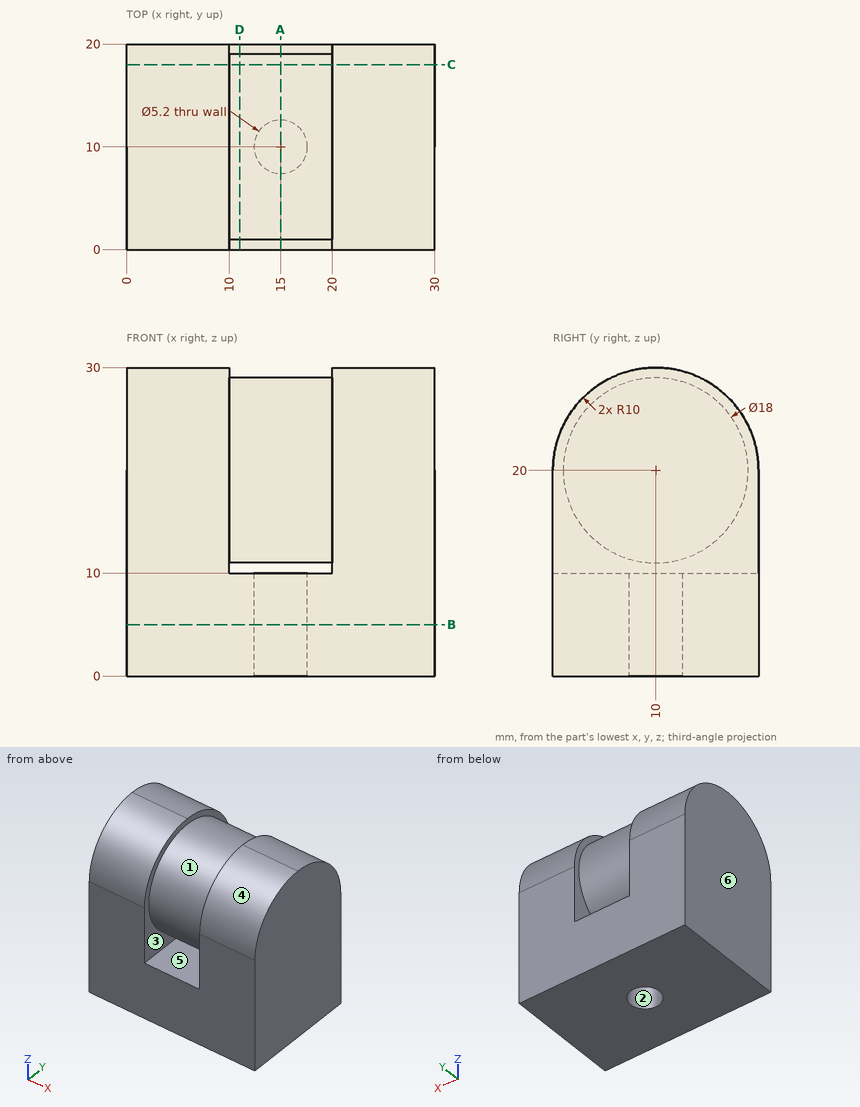
Answer from the drawing. Dimensions are ordinates in mm from the lowest x, y and z of the part. A direction names the side the tool comes from. Coordinates: 2 decimals unless noted, no trailing zeros. Order: outer loops, then holes, each group sorted by start corner. A loop starts at its lowest first (then second) coordinate and runs counter-clockwise, first axis right, second up. Notation, with made-up numbers: (46.5, 48) - (103.5, 48) arc R23 ccw to (103.5, 80) - close; hole circle Ø8 at (35.25, 6). An arc over 180 degrees is marked (long way). Use one line per item in the form item = value.
(1) Section D-D, the plane x = 11 is taken. Give the vertices of the cut face in (y, z), then the cut area to 3 significant figures.
Computed values:
outline = (0, 0) - (20, 0) - (20, 10) - (0, 10) - close; circle Ø18 at (10, 20)
area = 454 mm²
(2) Section C-C, the plane y = 18 is taken. Give the vertices of the cut face in (x, z), then the cut area to 3 significant figures.
Computed values:
outline = (0, 0) - (30, 0) - (30, 26) - (20, 26) - (20, 24.12) - (10, 24.12) - (10, 26) - (0, 26) - close; hole (10, 10) - (20, 10) - (20, 15.88) - (10, 15.88) - close
area = 702 mm²
(3) Section B-B, the plane z = 5 is taken. Give the vertices of the cut face in (x, y).
Computed values:
outline = (0, 0) - (30, 0) - (30, 20) - (0, 20) - close; hole circle Ø5.2 at (15, 10)
(4) Which of the six approach directions +Z, -Z, +X, -X, +Y, -Y give full straight-line access (tool end or side, diameter ignored) to the marked faces 5 and 6?
Computed values:
face_5 = +Y, -Y
face_6 = +Z, -Z, -X, +Y, -Y
(5) Section A-A, the plane x = 15 is taken. Give the vertices of the cut face in (y, z), then the cut area to 3 significant figures.
Computed values:
outline = (0, 0) - (7.4, 0) - (7.4, 10) - (0, 10) - close; circle Ø18 at (10, 20); (12.6, 0) - (20, 0) - (20, 10) - (12.6, 10) - close
area = 402 mm²
(6) Given pin 1 Ø3 at (x, y) = (15, 10) entering from +Z; pin 2 Ø2 at (x, y) = (12, 18) entering from +Z; pin 3 Ø3 at (x, y) = (13.5, 6.5) entering from +Z (3 decimals), each flat-ended and moving along its own axis, determine where each tip first touches the part or whether it passes through.
Computed values:
pin_1 = 29
pin_2 = 25.66
pin_3 = 28.775
(7) Straight lines are drawn through the part: L1, parallel to Y at x = 15, z = 2.25; L2, parallel to X at y = 5.75, z = 28.5; L3, parallel to Z at x = 11.75, y = 6.75. For each, find the intervals that lie inside material, in ascending order.
Computed values:
L1 = 0 to 7.4, 12.6 to 20
L2 = 0 to 10, 20 to 30
L3 = 0 to 10, 11.61 to 28.39
(8) For a pull along Z with two mould halves and no side action, classify the marked faces 1, 2, 3 and 4 as pulls with the +Z half, pulls with the -Z half, needs draft (parallel to the pull), parting line crosses it, or undercut.
Computed values:
face_1 = undercut
face_2 = needs draft
face_3 = undercut
face_4 = pulls with the +Z half
